Geometry: final body of the model. Coordinates: model frame, mm. A direction names the side the tool comes from. Coordinates: 2 decimals unless noted, no trailing zeros. Write each loop counter-clockwise with the first axis right and the second up, starting at its lowest first coordinate (ties: lowest second). Pieces come first, ordered by that corner, then holes. Notation, with made-up numbers: M 70,-5.75 L 90,-5.75 A19 ccw 90,20.25 Z; hole C -10,84.5 d3. An arc over 180 degrees is marked long. Write item = value, one per line. Start each with the question number.
Item 1: Ray query, L1, parallel to Z at x = 2.75, y = 3.75; L2, parallel to Y at x = -1.5, z = 0. Return the intervals inside material, ascending. Write a range as [from, to].
Item 2: Section D-D on x = 1. Output: boundary loops of the cut face in (y, z) (3 decimals).
Item 3: Reachability of faces 1 (the flat face through (0, 3, 0.25)), 2 (the flat face through (-2, 5.8, 0.5)), 3 (the flat face through (0, 6.075, 1)) from +Z, -Z, +X, -X, +Y, -Y: full face, straight path, thin tool, end or side. Return the list, or none.
Item 4: Section A-A on x = 0. Output: boundary loops of the cut face in (y, z) (3 decimals), plus the area to 3 significant figures.
Item 5: Pull-direction query (Y, two-part tool) for faces 4 (the cylindrical face through (0.19, -4.92, 0)), 5 (the flat face through (2, 5.8, 0.5)), 6 (the cylindrical face through (-0.54, 2.44, 0)); classes: +Y half, -Y half, draft (parallel to the pull), parting line (faces both ways), or undercut.
Item 6: Section C-C on z = 0.1. Output: boundary loops of the cut face in (x, y).
Item 7: Section B-B on y = 0. Output: boundary loops of the cut face in (x, z), plus the area to 3 significant figures.
Item 8: First-contact query: pin 1 Ø1.1 at (y, z) = (5.5, 0.5) entering from +X; pin 2 Ø0.7 at (y, z) = (5.5, 0.5) entering from -X; pin 3 Ø1.2 at (x, z) = (-1, 1) entering from -Y (3 decimals). Flat tips, straight axial feed; report the tip coordinate or a pass-through.
Autodesk Inventor part; units mm, degrees
ref_plane "YZ Plane" through (0, 0, 0) normal (1, 0, 0) x (0, 1, 0)
ref_plane "XZ Plane" through (0, 0, 0) normal (0, 1, 0) x (-1, 0, 0)
ref_plane "XY Plane" through (0, 0, 0) normal (0, 0, 1) x (1, 0, 0)
sketch "Szkic1" plane through (0, 0, 0) normal (0, 0, 1) x (1, 0, 0)
  circle A0 centre (0, 0) radius 2.5
  arc A1 (-2.1413, 4.4351) -> (2.1413, 4.4351) centre (0, 0) ccw
  line L0 (-2, 6.075) -> (2, 6.075)
  line L1 (-2, 6.075) -> (-2, 4.6603)
  line L2 (2, 6.075) -> (2, 4.6603)
  arc A2 (-2.1413, 4.4351) -> (-2, 4.6603) centre (-2.25, 4.6603) ccw
  arc A3 (2, 4.6603) -> (2.1413, 4.4351) centre (2.25, 4.6603) ccw
  point P0 (-2, 4.5006)
  point P1 (2, 4.5006)
  dimension "d0" = 5
  dimension "d1" = 9.85
  dimension "d3" = 4
  dimension "d4" = 0.25
extrude "Wyciągnięcie proste1" add sketch "Szkic1" along normal mid plane 0.5
sketch "Szkic2" plane through (0, 0, 0.25) normal (0, 0, 1) x (1, 0, 0)
  line L0 (2, 6.075) -> (-2, 6.075)
  line L1 (-2, 6.075) -> (2, 6.075)
  line L2 (2, 6.075) -> (2, 5.575)
  line L3 (2, 5.575) -> (-2, 5.575)
  line L4 (-2, 5.575) -> (-2, 6.075)
  dimension "d7" = 0.5
extrude "Wyciągnięcie proste2" add sketch "Szkic2" along normal blind 1.5
fillet "Zaokrąglenie1" radius 0.5 1 edges at (0, 6.075, -0.25)
properties part number "podkładka z jednym uchem" material "Stal"
Responses:
q1.L1 = [-0.25, 0.25]
q1.L2 = [-4.69, -2], [2, 6.01]
q2.outline = M -4.822,-0.25 L -2.291,-0.25 L -2.291,0.25 L -4.822,0.25 Z; M 2.291,-0.25 L 5.575,-0.25 A0.5 ccw 6.075,0.25 L 6.075,1.75 L 5.575,1.75 L 5.575,0.25 L 2.291,0.25 Z
q3.face_1 = +Z, +X, -X, -Y
q3.face_2 = +Z, -Z, -X, +Y
q3.face_3 = +Z, -Z, +X, -X, +Y
q4.outline = M -4.925,-0.25 L -2.5,-0.25 L -2.5,0.25 L -4.925,0.25 Z; M 2.5,-0.25 L 5.575,-0.25 A0.5 ccw 6.075,0.25 L 6.075,1.75 L 5.575,1.75 L 5.575,0.25 L 2.5,0.25 Z
q4.area = 3.70 mm²
q5.face_4 = parting line
q5.face_5 = draft
q5.face_6 = undercut
q6.outline = M -2.14,4.44 A4.92 ccw long 2.14,4.44 A0.25 cw 2,4.66 L 2,6.05 L -2,6.05 L -2,4.66 A0.25 cw Z; hole C 0,0 d5
q7.outline = M -4.92,-0.25 L -2.5,-0.25 L -2.5,0.25 L -4.92,0.25 Z; M 2.5,-0.25 L 4.92,-0.25 L 4.92,0.25 L 2.5,0.25 Z
q7.area = 2.42 mm²
q8.pin_1 = 2
q8.pin_2 = -2
q8.pin_3 = 5.575
